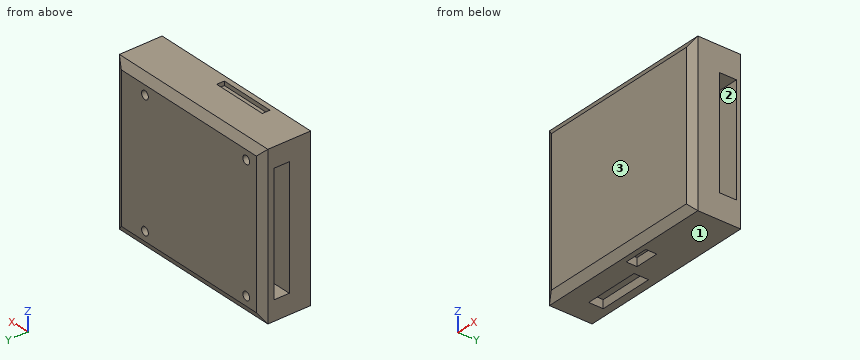
from build123d import *

# Parameters (mm, degrees)
SKETCH1_W             = 44
SKETCH1_H             = 38.5
BOSS_EXTRUDE1_DEPTH   = 12.7
CHAMFER1_SIZE         = 2
CHAMFER1_SIZE2        = 1.154700538
CHAMFER1_PART_2_SIZE  = 2
CHAMFER1_PART_2_SIZE2 = 1.154700538
SKETCH2_W             = 29
SKETCH2_H             = 3.71
CUT_EXTRUDE1_DEPTH    = 7.5
SKETCH3_W             = 26.5
SKETCH3_H             = 4.18
CUT_EXTRUDE2_DEPTH    = 7.5
SKETCH5_R             = 1
CUT_EXTRUDE3_DEPTH    = 2
SKETCH6_W             = 5.836145695
SKETCH6_H             = 2.652793498
SKETCH6_W_2           = 13.440820391
SKETCH6_H_2           = 3.537057997
CUT_EXTRUDE4_DEPTH    = 2
SKETCH7_W             = 13.529246841
SKETCH7_H             = 1.856955449
CUT_EXTRUDE5_DEPTH    = 1


with BuildPart() as part:
    # Sketch1 → Boss-Extrude1 (new body)
    with BuildSketch(Plane(origin=(0, 0, 0), x_dir=(1, 0, 0), z_dir=(0, 1, 0))):
        Rectangle(SKETCH1_W, SKETCH1_H)
    extrude(amount=BOSS_EXTRUDE1_DEPTH)

    # Chamfer1
    chamfer1_edges = [part.edges().sort_by_distance(p)[0] for p in [
        (-22, 12.7, 0),
        (0, 12.7, 19.25),
        (22, 12.7, 0),
        (0, 12.7, -19.25),
    ]]
    chamfer1_side = [part.faces().sort_by_distance(p)[0] for p in [
        (0, 12.7, 0),
    ]]
    chamfer(chamfer1_edges, length=CHAMFER1_SIZE, length2=CHAMFER1_SIZE2, reference=chamfer1_side[0])

    # Chamfer1 part 2
    chamfer1_part_2_edges = [part.edges().sort_by_distance(p)[0] for p in [
        (0, 0, 19.25),
        (-22, 0, 0),
        (0, 0, -19.25),
        (22, 0, 0),
    ]]
    chamfer1_part_2_side = [part.faces().sort_by_distance(p)[0] for p in [
        (0, 0, 0),
    ]]
    chamfer(chamfer1_part_2_edges, length=CHAMFER1_PART_2_SIZE, length2=CHAMFER1_PART_2_SIZE2, reference=chamfer1_part_2_side[0])

    # Sketch2 → Cut-Extrude1 (cut)
    with BuildSketch(Plane.ZY.offset(22)):
        with Locations((0, 8.205)):
            Rectangle(SKETCH2_W, SKETCH2_H)
    extrude(amount=-CUT_EXTRUDE1_DEPTH, mode=Mode.SUBTRACT)

    # Sketch3 → Cut-Extrude2 (cut)
    with BuildSketch(Plane(origin=(22, 0, 0), x_dir=(0, 0, -1), z_dir=(1, 0, 0))):
        with Locations((0, 8.44)):
            Rectangle(SKETCH3_W, SKETCH3_H)
    extrude(amount=-CUT_EXTRUDE2_DEPTH, mode=Mode.SUBTRACT)

    # Sketch5 → Cut-Extrude3 (cut)
    with BuildSketch(Plane(origin=(0, 12.7, 0), x_dir=(1, 0, 0), z_dir=(0, 1, 0))):
        with Locations((-17, -15)):
            Circle(SKETCH5_R)
        with Locations((-17, 15)):
            Circle(SKETCH5_R)
        with Locations((13, 15)):
            Circle(SKETCH5_R)
        with Locations((13, -15)):
            Circle(SKETCH5_R)
    extrude(amount=-CUT_EXTRUDE3_DEPTH, mode=Mode.SUBTRACT)

    # Sketch6 → Cut-Extrude4 (cut)
    with BuildSketch(Plane(origin=(0, 0, -19.25), x_dir=(-1, 0, 0), z_dir=(0, 0, -1))):
        with Locations((-2.166448024, 3.719313114)):
            Rectangle(SKETCH6_W, SKETCH6_H)
        with Locations((9.726909494, 7.919569487)):
            Rectangle(SKETCH6_W_2, SKETCH6_H_2)
    extrude(amount=-CUT_EXTRUDE4_DEPTH, mode=Mode.SUBTRACT)

    # Sketch7 → Cut-Extrude5 (cut)
    with BuildSketch(Plane.XY.offset(19.25)):
        with Locations((-4.642388622, 3.277180865)):
            Rectangle(SKETCH7_W, SKETCH7_H)
    extrude(amount=-CUT_EXTRUDE5_DEPTH, mode=Mode.SUBTRACT)


solid = part.part
For this review, take the finished solid that the model builds, in its own axes (mm). Face numbers are marked on the shaded views. Coordinates: 2 decimals unless noted, no trailing zeros. Loops run counter-clockwise (first coordinate to the right, second up) from the corner with the lowest first, then second, coordinate; pieces in that order, holes last. Notation, with made-up numbers: (21.5, 10.25) - (39.5, 10.25) arc R25 ccw to (39.5, 42.25) - close; hole circle Ø11 at (-8, 35.5). An arc over 180 degrees is marked (long way). Use a Markdown table: item, result. Add a question column.
Item 1: We need section D-D (x = -17). Give the boundary of the cut face in (y, z).
Item 2: We need section B-B (z = 5.5). Give the boundary of the cut face in (x, y), and give its area (3 significant figures).
Item 3: For line 1 (X direction, y = 11.45, z = -15); line 2 (Z direction, x = -17, y = 11.55); line 3 (Y direction, x = -15.5, z = 7), list the stretches that pass through material, from the lowest coordinate up.
Item 4: We need section A-A (x = 15). Give the boundary of the cut face in (y, z), and give its area (3 significant figures).
Item 5: Mouldability with a two-part tool opening along Z and no side actions: class the marked faces 1, 2 and 3 as pulls with the +Z half, pulls with the -Z half, needs draft (parallel to the pull), parting line crosses it, or undercut.
Item 6: We need section C-C (y = 7.25). Give the boundary of the cut face in (x, z), and give its area (3 significant figures).
Item 7: Insertion check: pin 1 Ø0.6 at (x, z) = (-10, -18) entering from -Y; pin 2 Ø0.9 at (x, y) = (-4, 3.5) entering from +Z. Each pin has a flat end and moves straight along its axis. Give the tip position at first contact, or say it passes through.
Results list:
| question | item | result |
|---|---|---|
| 1 | outline | (0, -17.25) - (1.15, -19.25) - (11.55, -19.25) - (12.7, -17.25) - (12.7, -16) - (10.7, -16) - (10.7, -14) - (12.7, -14) - (12.7, 14) - (10.7, 14) - (10.7, 16) - (12.7, 16) - (12.7, 17.25) - (11.55, 19.25) - (1.15, 19.25) - (0, 17.25) - close; hole (6.35, -14.5) - (10.06, -14.5) - (10.06, 14.5) - (6.35, 14.5) - close |
| 2 | outline | (-22, 1.15) - (-20, 0) - (20, 0) - (22, 1.15) - (22, 6.35) - (14.5, 6.35) - (14.5, 10.53) - (22, 10.53) - (22, 11.55) - (20, 12.7) - (-20, 12.7) - (-22, 11.55) - (-22, 10.06) - (-14.5, 10.06) - (-14.5, 6.35) - (-22, 6.35) - close |
| 2 | area | 495 mm^2 |
| 3 | line 1 | x = -22 to -18, -16 to 12, 14 to 22 |
| 3 | line 2 | z = -19.24 to -16, -14 to 14, 16 to 19.24 |
| 3 | line 3 | y = 0 to 6.35, 10.06 to 12.7 |
| 4 | outline | (0, -17.25) - (1.15, -19.25) - (11.55, -19.25) - (12.7, -17.25) - (12.7, 17.25) - (11.55, 19.25) - (1.15, 19.25) - (0, 17.25) - close; hole (6.35, -13.25) - (10.53, -13.25) - (10.53, 13.25) - (6.35, 13.25) - close |
| 4 | area | 374 mm^2 |
| 5 | face 1 | pulls with the -Z half |
| 5 | face 2 | undercut |
| 5 | face 3 | needs draft |
| 6 | outline | (-22, -19.25) - (-16.45, -19.25) - (-16.45, -17.25) - (-3.01, -17.25) - (-3.01, -19.25) - (22, -19.25) - (22, -13.25) - (14.5, -13.25) - (14.5, 13.25) - (22, 13.25) - (22, 19.25) - (-22, 19.25) - (-22, 14.5) - (-14.5, 14.5) - (-14.5, -14.5) - (-22, -14.5) - close |
| 6 | area | 1,250 mm^2 |
| 7 | pin 1 | stops at y = 0.26 |
| 7 | pin 2 | stops at z = 18.25 |
